The listing builds one solid part. Answer for the finished solid, in the listing's coordinates (mm). Face numbers are marked on the shaded views. A direction names the side the tool comes from. Round coordinates to 2 decimals unless told otherwise and drop trailing zeros. Loops run counter-clockwise (first coordinate to the right, second up) from the corner with the lowest first, then second, coordinate; pieces in that order, holes last. Notation, with made-up numbers: M -19,21 L 32,21 A12 ccw 32,28 Z; hole C 67.25,-7 d2. An arc over 180 degrees is marked long. Answer as a JSON object with one key per item and string values.
```python
from build123d import *

# Parameters (mm, degrees)
F0_W     = 30
F0_H     = 10
F1_DEPTH = 40
F2_W     = 25
F2_H     = 10
F3_DEPTH = 12
F4_W     = 25
F4_H     = 10
F5_DEPTH = 7


with BuildPart() as f1:
    # F0 (on Top) → F1 (new body)
    with BuildSketch(Plane.XY):
        Rectangle(F0_W, F0_H)
    extrude(amount=F1_DEPTH)

    # F2 (on face) → F3 (join)
    with BuildSketch(Plane.XY.offset(40)):
        Rectangle(F2_W, F2_H)
    extrude(amount=F3_DEPTH)

    # F4 (on face) → F5 (join)
    with BuildSketch(Plane.XY.offset(52)):
        Rectangle(F4_W, F4_H)
    extrude(amount=F5_DEPTH)


solid = f1.part
```
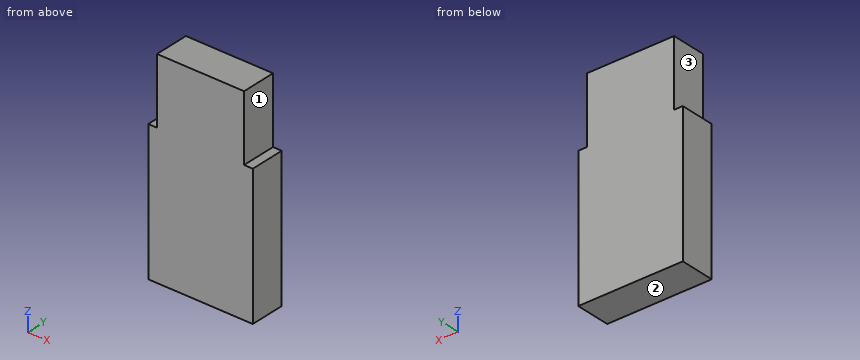
Item 1: Flat-ended cylindrical pins translate along their axes: P1, Ø2, axis at x = -14, y = 2, coming from the +Z side; P2, Ø3, axis at y = 2.5, z = 49.5, coming from the +X side. Find the tip coordinate at first contact, or state that the pin passes through.
Values follow:
{"P1": "z = 40", "P2": "x = 12.5"}
Item 2: Which of the six approach directions +Z, -Z, +X, -X, +Y, -Y give full straight-line access (tool end or side, diameter ignored) to the marked faces 1, 2 and 3?
Values follow:
{"face 1": "+Z, +X, +Y, -Y", "face 2": "-Z, +X, -X, +Y, -Y", "face 3": "+Z, -X, +Y, -Y"}
Item 3: The part is cut by section A-A (y = 0.75). Give the vertices of the cut face in (x, z).
Values follow:
{"outline": "M -15,0 L 15,0 L 15,40 L 12.5,40 L 12.5,59 L -12.5,59 L -12.5,40 L -15,40 Z"}
Item 4: Straight lines are drawn through the part: line 1 (X direction, y = 2, z = 43); line 2 (Z direction, x = 13.75, y = -1). For each, find the intervals that lie inside material, in ascending order.
Values follow:
{"line 1": "-12.5 to 12.5", "line 2": "0 to 40"}
Item 5: The part is cut by section B-B (z = 45.5). Give the vertices of the cut face in (x, y), then the cut area to 3 significant figures.
Values follow:
{"outline": "M -12.5,-5 L 12.5,-5 L 12.5,5 L -12.5,5 Z", "area": "250 mm^2"}
